Work out the finished part from the listing and answer in its coordinate system (mm). A direction names the side the tool comes from. Coordinates: 2 decimals unless noted, no trailing zeros. Write each loop counter-clockwise with the first axis right and the second up, starting at its lowest first coordinate (ties: lowest second). Pieces come first, ordered by that corner, then holes. Notation, with made-up numbers: (66, 18) - (121, 18) arc R20 cw to (121, 57) - close; hole circle Ø5 at (68.5, 28). An arc over 180 degrees is marked (long way). One line per item, written item: value.
```python
from build123d import *

# Parameters (mm, degrees)
BOSS_EXTRUDE1_DEPTH = 18.5
BOSS_EXTRUDE2_DEPTH = 3
BOSS_EXTRUDE3_START = 7
BOSS_EXTRUDE3_DEPTH = 3.5
SKETCH4_W           = 6.5
SKETCH4_H           = 2.25
BOSS_EXTRUDE4_DEPTH = 20
FILLET1_R           = 2.25
BOSS_EXTRUDE5_DEPTH = 7
BOSS_EXTRUDE6_DEPTH = 3
SKETCH7_R           = 2.5
CUT_EXTRUDE1_DEPTH  = 73.232264259
SKETCH8_R           = 2.2
CUT_EXTRUDE2_DEPTH  = 71.763691255
CUT_EXTRUDE3_REACH  = 72.764
SKETCH9_R           = 2.2
BOSS_EXTRUDE7_REACH = 74.907
SKETCH10_R          = 3.5
SKETCH10_R_2        = 2.5
BOSS_EXTRUDE8_REACH = 72.039
SKETCH11_R          = 3.5
SKETCH11_R_2        = 2.5
CUT_EXTRUDE4_REACH  = 66.742
SKETCH12_W          = 7
SKETCH12_H          = 5


with BuildPart() as part:
    # Sketch1 → Boss-Extrude1 (new body)
    with BuildSketch(Plane(origin=(0, 0, 0), x_dir=(1, 0, 0), z_dir=(0, 1, 0))):
        Polygon((40.5, 0), (0, 0), (0, -55), (3, -55), (3, -3), (40.5, -3), align=None)
    extrude(amount=BOSS_EXTRUDE1_DEPTH)

    # Sketch2 → Boss-Extrude2 (add)
    with BuildSketch(Plane.XZ):
        with BuildLine():
            Line((40.5, 3), (23.5, 19.5))
            Line((23.5, 19.5), (23.5, 37))
            ThreePointArc((23.5, 37), (20.571067812, 44.071067812), (13.5, 47))
            Line((13.5, 47), (3, 47))
            Line((3, 47), (3, 3))
            Line((3, 3), (40.5, 3))
        make_face()
    extrude(amount=-BOSS_EXTRUDE2_DEPTH)

    # Sketch3 → Boss-Extrude3 (add)
    with BuildSketch(Plane(origin=(0, 3, 0), x_dir=(1, 0, 0), z_dir=(0, 1, 0)).offset(BOSS_EXTRUDE3_START)):
        with BuildLine():
            Line((3, -47), (13.5, -47))
            ThreePointArc((13.5, -47), (23.5, -37), (13.5, -27))
            Line((13.5, -27), (3, -27))
            Line((3, -27), (3, -47))
        make_face()
    extrude(amount=BOSS_EXTRUDE3_DEPTH)

    # Sketch4 → Boss-Extrude4 (add)
    with BuildSketch(Plane.XY.offset(47)):
        with Locations((6.25, 14.625)):
            Rectangle(SKETCH4_W, SKETCH4_H)
    extrude(amount=-BOSS_EXTRUDE4_DEPTH)

    # Fillet1
    fillet1_edges = [part.edges().sort_by_distance(p)[0] for p in [
        (9.5, 15.75, 37),
    ]]
    fillet(fillet1_edges, radius=FILLET1_R - 0.0001)  # a hair under: the kernel refuses the full size

    # Sketch5 → Boss-Extrude5 (add)
    with BuildSketch(Plane.XZ):
        Polygon((0, 28.5), (0, 8.5), (9, 8.5), (9, 10.5), (3, 10.5), (3, 28.5), align=None)
    extrude(amount=BOSS_EXTRUDE5_DEPTH)

    # Sketch6 → Boss-Extrude6 (add)
    with BuildSketch(Plane.XZ.offset(7)):
        with BuildLine():
            Line((0, 8.5), (0, 28.5))
            Line((0, 28.5), (13.5, 28.5))
            ThreePointArc((13.5, 28.5), (23.5, 18.5), (13.5, 8.5))
            Line((13.5, 8.5), (0, 8.5))
        make_face()
    extrude(amount=BOSS_EXTRUDE6_DEPTH)

    # Sketch7 → Cut-Extrude1 (cut, through all)
    with BuildSketch(Plane(origin=(0, 13.5, 0), x_dir=(1, 0, 0), z_dir=(0, 1, 0))):
        with Locations(Location((15.5, -21.5, 0), (0, 0, 270))):
            Circle(SKETCH7_R)
        with Locations(Location((15.5, -37, 0), (0, 0, 270))):
            Circle(SKETCH7_R)
    extrude(amount=-CUT_EXTRUDE1_DEPTH, mode=Mode.SUBTRACT)

    # Sketch8 → Cut-Extrude2 (cut, through all)
    with BuildSketch(Plane.ZY):
        with Locations((11, 8.5)):
            Circle(SKETCH8_R)
        with Locations((51.5, 8.5)):
            Circle(SKETCH8_R)
    extrude(amount=-CUT_EXTRUDE2_DEPTH, mode=Mode.SUBTRACT)

    # Sketch9 → Cut-Extrude3 (cut, up to next)
    with BuildSketch(Plane(origin=(0, 0, 0), x_dir=(-1, 0, 0), z_dir=(0, 0, -1)), mode=Mode.PRIVATE) as cut_extrude3_sk1:
        with Locations((-34.5, 8.5)):
            Circle(SKETCH9_R)
    cut_extrude3_tool1 = extrude(cut_extrude3_sk1.sketch, amount=-CUT_EXTRUDE3_REACH, mode=Mode.PRIVATE) & part.part
    # Sketch9 → Cut-Extrude3 (cut, up to next)
    with BuildSketch(Plane(origin=(0, 0, 0), x_dir=(-1, 0, 0), z_dir=(0, 0, -1)), mode=Mode.PRIVATE) as cut_extrude3_sk2:
        with Locations((-15, 8.5)):
            Circle(SKETCH9_R)
    cut_extrude3_tool2 = extrude(cut_extrude3_sk2.sketch, amount=-CUT_EXTRUDE3_REACH, mode=Mode.PRIVATE) & part.part
    add(cut_extrude3_tool1.solids().sort_by_distance((34.5, 8.5, 0))[0], mode=Mode.SUBTRACT)
    add(cut_extrude3_tool2.solids().sort_by_distance((15, 8.5, 0))[0], mode=Mode.SUBTRACT)

    # Sketch10 → Boss-Extrude7 (add, up to next)
    with BuildSketch(Plane(origin=(0, -7, 0), x_dir=(1, 0, 0), z_dir=(0, 1, 0)), mode=Mode.PRIVATE) as boss_extrude7_sk1:
        with Locations(Location((15.5, -21.5, 0), (0, 0, 270))):
            Circle(SKETCH10_R)
        with Locations(Location((15.5, -21.5, 0), (0, 0, 270))):
            Circle(SKETCH10_R_2, mode=Mode.SUBTRACT)
    boss_extrude7_tool1 = extrude(boss_extrude7_sk1.sketch, amount=BOSS_EXTRUDE7_REACH, mode=Mode.PRIVATE) - part.part
    add(boss_extrude7_tool1.solids().sort_by_distance((15.5, -7, 18.098995))[0])

    # Sketch11 → Boss-Extrude8 (add, up to next)
    with BuildSketch(Plane(origin=(0, 3, 0), x_dir=(1, 0, 0), z_dir=(0, 1, 0)), mode=Mode.PRIVATE) as boss_extrude8_sk1:
        with Locations(Location((15.5, -37, 0), (0, 0, 90))):
            Circle(SKETCH11_R)
        with Locations(Location((15.5, -37, 0), (0, 0, 270))):
            Circle(SKETCH11_R_2, mode=Mode.SUBTRACT)
    boss_extrude8_tool1 = extrude(boss_extrude8_sk1.sketch, amount=BOSS_EXTRUDE8_REACH, mode=Mode.PRIVATE) - part.part
    add(boss_extrude8_tool1.solids().sort_by_distance((15.5, 3, 40.401005))[0])

    # Cut-Extrude4: up to this face of the body (flat: up to its plane)
    cut_extrude4_end = Plane(part.part.faces().sort_by_distance((21.584376674, 10.874217494, 3))[0])
    # Sketch12 → Cut-Extrude4 (cut, up to the picked face)
    with BuildSketch(Plane.XY.offset(47), mode=Mode.PRIVATE) as cut_extrude4_sk1:
        with Locations((15.5, -3.5)):
            Rectangle(SKETCH12_W, SKETCH12_H)
    cut_extrude4_tool1 = split(extrude(cut_extrude4_sk1.sketch, amount=-CUT_EXTRUDE4_REACH, mode=Mode.PRIVATE), bisect_by=cut_extrude4_end, keep=Keep.BOTH, mode=Mode.PRIVATE)
    # Sketch12 → Cut-Extrude4 (cut, up to the picked face)
    with BuildSketch(Plane.XY.offset(47), mode=Mode.PRIVATE) as cut_extrude4_sk2:
        with Locations((15.5, 6.5)):
            Rectangle(SKETCH12_W, SKETCH12_H)
    cut_extrude4_tool2 = split(extrude(cut_extrude4_sk2.sketch, amount=-CUT_EXTRUDE4_REACH, mode=Mode.PRIVATE), bisect_by=cut_extrude4_end, keep=Keep.BOTH, mode=Mode.PRIVATE)
    add(cut_extrude4_tool1.solids().sort_by(Axis((15.5, -3.5, 47), (0, 0, -1)))[0], mode=Mode.SUBTRACT)
    add(cut_extrude4_tool2.solids().sort_by(Axis((15.5, 6.5, 47), (0, 0, -1)))[0], mode=Mode.SUBTRACT)


solid = part.part
```
Item 1: Consider probe 1 along X at (y, z) = (3.1, 37); probe 2 along X at (y, z) = (1.05, 37); probe 3 along Y at (x, z) = (4.5, 34.5). Determine where each line is inside the solid, lowest interval first.
Evaluation:
probe 1: x = 0 to 3, 12 to 13, 18 to 19
probe 2: x = 0 to 13, 18 to 23.5
probe 3: y = 0 to 3, 10 to 15.75
Item 2: Determine the mould class of faces 5 (the face through (32.119, 1.479, 11.135)), 6 (the face through (8.86, 15.07, 36.86)), 7 (the face through (1.479, 10.355, 12.183)) for opening direction Y: +Y half, -Y half, draft (parallel to the pull), parting line (faces both ways), or undercut.
Evaluation:
face 5: draft
face 6: +Y half
face 7: undercut
Item 3: Section C-C, the plane y = 7 is taken. Determine the outline of the cut face in (x, z).
Evaluation:
outline: (0, 0) - (13.39, 0) - (13.39, 3) - (3, 3) - (3, 9.39) - (0, 9.39) - close; (0, 12.61) - (3, 12.61) - (3, 49.89) - (0, 49.89) - close; (0, 53.11) - (3, 53.11) - (3, 55) - (0, 55) - close; (16.61, 0) - (32.89, 0) - (32.89, 3) - (16.61, 3) - close; (36.11, 0) - (40.5, 0) - (40.5, 3) - (36.11, 3) - close
Item 4: Which of the six approach directions +Z, -Z, +X, -X, +Y, -Y give full straight-line access (tool end or side, diameter ignored) to faces 1 (the face through (18, -6, 20)), 2 (the face through (23.5, 1, 28)), 3 (the face through (23.5, -8.5, 18.7)), 4 (the face through (11, 10, 37))?
Evaluation:
face 1: +Z, -Z, +X
face 2: +Z, +X, +Y, -Y
face 3: +X, -Y
face 4: none
Item 5: Section B-B, the plane x = 4 is taken. Determine the outline of the cut face in (y, z), then the cut area to 4 significant figures.
Evaluation:
outline: (-10, 8.5) - (0, 8.5) - (0, 0) - (18.5, 0) - (18.5, 3) - (3, 3) - (3, 47) - (0, 47) - (0, 10.5) - (-7, 10.5) - (-7, 28.5) - (-10, 28.5) - close; (10, 27) - (15.75, 27) - (15.75, 47) - (10, 47) - close
area: 376.5 mm2
Item 6: Section D-D, the plane z = 21.5 is taken. Determine the outline of the cut face in (x, y).
Evaluation:
outline: (0, -10) - (13, -10) - (13, -6) - (12, -6) - (12, -7) - (3, -7) - (3, 0) - (12, 0) - (12, -1) - (13, -1) - (13, 3) - (3, 3) - (3, 18.5) - (0, 18.5) - close; (18, -10) - (23.04, -10) - (23.04, -7) - (19, -7) - (19, -6) - (18, -6) - close; (18, -1) - (19, -1) - (19, 0) - (23.5, 0) - (23.5, 3) - (18, 3) - close
Item 7: Given pin 1 (3.5 mm diameter, centred on x = 16, z = 35.5, fed in from +Y); pin 2 (6 mm diameter, centred on x = 15.5, z = 21.5, fed in from +Y); pin 3 (0.9 mm diameter, centred on x = 7, y = 2, fed in from +Z), each flat-ended and moving along its own axis, determine where each tip first touches the part or whether it passes through.
Evaluation:
pin 1: stops at y = 13.5
pin 2: stops at y = 3
pin 3: stops at z = 47
Item 8: Section A-A, the plane z = 51.5 is taken. Determine the outline of the cut face in (x, y), then the cut area to 3 significant figures.
Evaluation:
outline: (0, 0) - (3, 0) - (3, 6.3) - (0, 6.3) - close; (0, 10.7) - (3, 10.7) - (3, 18.5) - (0, 18.5) - close
area: 42.3 mm2
